```python
from build123d import *

# Parameters (mm, degrees)
AUFSATZ_LINEAR_AUSTRAGEN1_DEPTH = 54
SCHNITT_LINEAR_AUSTRAGEN1_DEPTH = 7
SCHNITT_LINEAR_AUSTRAGEN2_DEPTH = 7
SCHNITT_LINEAR_AUSTRAGEN3_REACH = 83
SKIZZE4_R                       = 4.5
SKIZZE5_R                       = 7.5
SCHNITT_LINEAR_AUSTRAGEN4_DEPTH = 8


with BuildPart() as part:
    # Skizze1 → Aufsatz-Linear austragen1 (new body)
    with BuildSketch(Plane.XY):
        Polygon((0, 6), (0, 0), (83.5, 0), (83.5, 14.5), (81, 14.5), (81, 32.5), (83.5, 32.5), (83.5, 35.5), (68.5, 35.5), (65.5, 32.5), (65.5, 11), (60.5, 6), align=None)
    extrude(amount=AUFSATZ_LINEAR_AUSTRAGEN1_DEPTH)

    # Skizze2 → Schnitt-Linear austragen1 (cut, through all)
    with BuildSketch(Plane(origin=(0, 6, 0), x_dir=(1, 0, 0), z_dir=(0, 1, 0))):
        Polygon((28.521103298, -54), (0, -4.6), (0, -54), align=None)
    extrude(amount=-SCHNITT_LINEAR_AUSTRAGEN1_DEPTH, mode=Mode.SUBTRACT)

    # Skizze3 → Schnitt-Linear austragen2 (cut, through all)
    with BuildSketch(Plane(origin=(0, 6, 0), x_dir=(1, 0, 0), z_dir=(0, 1, 0))):
        Polygon((14, -5.452863896), (14, -7), (18, -7), (18, -5.459056191), (27.455362685, 0), (4.555362685, 0), align=None)
    extrude(amount=-SCHNITT_LINEAR_AUSTRAGEN2_DEPTH, mode=Mode.SUBTRACT)

    # Skizze4 → Schnitt-Linear austragen3 (cut, up to next)
    with BuildSketch(Plane(origin=(81, 0, 0), x_dir=(0, 0, -1), z_dir=(1, 0, 0)), mode=Mode.PRIVATE) as schnitt_linear_austragen3_sk1:
        with Locations((-9.5, 23.5)):
            Circle(SKIZZE4_R)
    schnitt_linear_austragen3_tool1 = extrude(schnitt_linear_austragen3_sk1.sketch, amount=-SCHNITT_LINEAR_AUSTRAGEN3_REACH, mode=Mode.PRIVATE) & part.part
    add(schnitt_linear_austragen3_tool1.solids().sort_by_distance((81, 23.5, 9.5))[0], mode=Mode.SUBTRACT)
    # Skizze4 → Schnitt-Linear austragen3 (cut, up to next)
    with BuildSketch(Plane(origin=(81, 0, 0), x_dir=(0, 0, -1), z_dir=(1, 0, 0)), mode=Mode.PRIVATE) as schnitt_linear_austragen3_sk2:
        with Locations((-43.5, 23.5)):
            Circle(SKIZZE4_R)
    schnitt_linear_austragen3_tool2 = extrude(schnitt_linear_austragen3_sk2.sketch, amount=-SCHNITT_LINEAR_AUSTRAGEN3_REACH, mode=Mode.PRIVATE) & part.part
    add(schnitt_linear_austragen3_tool2.solids().sort_by_distance((81, 23.5, 43.5))[0], mode=Mode.SUBTRACT)

    # Skizze5 → Schnitt-Linear austragen4 (cut)
    with BuildSketch(Plane.ZY.offset(-65.5)):
        with Locations((43.5, 23.5)):
            Circle(SKIZZE5_R)
        with Locations((9.5, 23.5)):
            Circle(SKIZZE5_R)
    extrude(amount=-SCHNITT_LINEAR_AUSTRAGEN4_DEPTH, mode=Mode.SUBTRACT)


solid = part.part
```
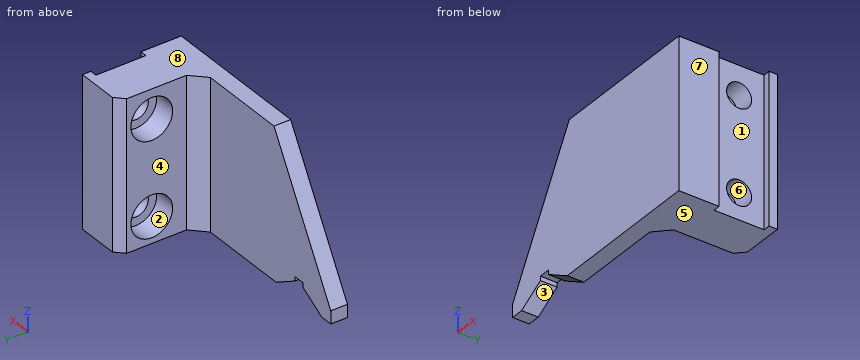
Here's how the part is built. I have some questions about the finished solid (model axes, mm). Face numbers are marked on the shaded views. A direction names the side the tool comes from. Coordinates: 2 decimals unless noted, no trailing zeros. Order: outer loops, then holes, each group sorted by start corner. A loop starts at its lowest first (then second) coordinate and runs counter-clockwise, first axis right, second up.
1) I need wall thicknesses on line 1 (Y direction, x = 70.5, z = 9.5); line 2 (X direction, y = 14, z = 15); line 3 (X direction, y = 27, z = 38). Which ranges of each line are inside material? Lowest first, please.
2) Imagine slicing it at B-B on z = 9.5. List the corners of the cut face in (x, y) for me, and give its area (3 significant figures).
3) Will these pins go through, and if not, where does the flat tip stop? pin 1 (16.5 mm diameter, centred on y = 23, z = 7, fed in from -X); pin 2 (4.5 mm diameter, centred on y = 23.5, z = 43, fed in from -X) (1 decimal); pin 3 (13.5 mm diameter, centred on y = 23.5, z = 43.5, fed in from +X); pin 4 (2 mm diameter, centred on x = 15.5, y = 2, fed in from -Z).
4) Which directions (+Z, -Z, +X, -X, +Y, -Y) give clear straight access to the entire face, cutting with the end or side of a thin tool? Please do the marked faces 1, 2, 3 and 4.
5) Imagine slicing it at C-C on x = 70. List the corners of the cut face in (y, z) for me.
6) Imagine slicing it at D-D on z = 37. List the corners of the cut face in (x, y) for me, and give its area (3 significant figures).
7) We'd pull the mould along Z, two halves only. Please class the marked faces 5, 6, 7 and 8: +Z half, -Z half, draft (parallel to the pull), parting line (faces both ways), or undercut.
8) Imagine slicing it at A-A on y = 23.5. List the corners of the cut face in (x, z) for me.
Response values:
1. line 1: y = 0 to 16, 31 to 35.5
1. line 2: x = 65.5 to 83.5
1. line 3: x = 73.5 to 81
2. outline: (2.83, 0) - (83.5, 0) - (83.5, 14.5) - (81, 14.5) - (81, 19) - (73.5, 19) - (73.5, 16) - (65.5, 16) - (65.5, 11) - (60.5, 6) - (2.83, 6) - close; (65.5, 31) - (73.5, 31) - (73.5, 28) - (81, 28) - (81, 32.5) - (83.5, 32.5) - (83.5, 35.5) - (68.5, 35.5) - (65.5, 32.5) - close
2. area: 791 mm2
3. pin 1: stops at x = 65.5
3. pin 2: passes through
3. pin 3: stops at x = 81
3. pin 4: stops at z = 7
4. face 1: +Z, -Z, +X
4. face 2: -X
4. face 3: -Z, +Y, -Y
4. face 4: +Z, -Z, -X, +Y
5. outline: (0, 0) - (35.5, 0) - (35.5, 54) - (0, 54) - close; hole circle Ø15 at (23.5, 9.5); hole circle Ø15 at (23.5, 43.5)
6. outline: (18.71, 0) - (83.5, 0) - (83.5, 14.5) - (81, 14.5) - (81, 32.5) - (83.5, 32.5) - (83.5, 35.5) - (68.5, 35.5) - (65.5, 32.5) - (65.5, 27.24) - (73.5, 27.24) - (73.5, 19.76) - (65.5, 19.76) - (65.5, 11) - (60.5, 6) - (18.71, 6) - close
6. area: 823 mm2
7. face 5: -Z half
7. face 6: undercut
7. face 7: draft
7. face 8: +Z half
8. outline: (65.5, 0) - (81, 0) - (81, 5) - (73.5, 5) - (73.5, 2) - (65.5, 2) - close; (65.5, 17) - (73.5, 17) - (73.5, 14) - (81, 14) - (81, 39) - (73.5, 39) - (73.5, 36) - (65.5, 36) - close; (65.5, 51) - (73.5, 51) - (73.5, 48) - (81, 48) - (81, 54) - (65.5, 54) - close
